Build history of the part. All positions in model axes, mm. A direction names the side the tool comes from. Give positions to 0.01 mm unless a question says otherwise; leave off trailing zeros. Loops run counter-clockwise (first coordinate to the right, second up) from the corner with the lowest first, then second, coordinate; pieces in that order, holes last. Notation, with made-up numbers: (78, 73) -> (106, 73) arc R26 ccw to (106, 96) -> close; hole circle Ø6 at (-29.75, -15.5). An arc over 180 degrees is marked (long way). Answer as a JSON object with one key per item and string values. Group by question number.
from build123d import *

# Parameters (mm, degrees)
SKETCH1_R           = 3
BOSS_EXTRUDE1_DEPTH = 7.5
SKETCH2_W           = 9
SKETCH2_H           = 5
CUT_EXTRUDE1_DEPTH  = 4.5
SKETCH3_W           = 5
SKETCH3_H           = 5
CUT_EXTRUDE2_DEPTH  = 1.5
CUT_EXTRUDE3_DEPTH  = 6


with BuildPart() as part:
    # Sketch1 → Boss-Extrude1 (new body)
    with BuildSketch(Plane.XY):
        with BuildLine():
            Line((-1.5, 5), (-3.5, 5))
            ThreePointArc((-3.5, 5), (-8.5, 0), (-3.5, -5))
            Line((-3.5, -5), (3.5, -5))
            Line((3.5, -5), (3.5, 5))
            Line((3.5, 5), (2.5, 5))
            Line((2.5, 5), (2.5, 4))
            Line((2.5, 4), (-1.5, 4))
            Line((-1.5, 4), (-1.5, 5))
        make_face()
        with Locations((-3.5, 0)):
            Circle(SKETCH1_R, mode=Mode.SUBTRACT)
    extrude(amount=BOSS_EXTRUDE1_DEPTH)

    # Sketch2 → Cut-Extrude1 (cut)
    with BuildSketch(Plane.XY.offset(7.5)):
        with Locations((-4, 2.5)):
            Rectangle(SKETCH2_W, SKETCH2_H)
    extrude(amount=-CUT_EXTRUDE1_DEPTH, mode=Mode.SUBTRACT)

    # Sketch3 → Cut-Extrude2 (cut)
    with BuildSketch(Plane.XY.offset(7.5)):
        with Locations((-6, -2.5)):
            Rectangle(SKETCH3_W, SKETCH3_H)
    extrude(amount=-CUT_EXTRUDE2_DEPTH, mode=Mode.SUBTRACT)

    # Sketch4 → Cut-Extrude3 (cut)
    with BuildSketch(Plane(origin=(0, 5, 0), x_dir=(1, 0, 0), z_dir=(0, 1, 0))):
        Polygon((3.5, -6.5), (2.5, -6.5), (0.5, -3), (0.5, -7.5), (3.5, -7.5), align=None)
    extrude(amount=-CUT_EXTRUDE3_DEPTH, mode=Mode.SUBTRACT)


solid = part.part
(1) Probe line 1 along X through (y, z) = (0, 2.5); line 2 along Z through (x, y) = (-2, 4); line 3 along Z through (x, y) = (-5, -3.5). List the from-to ranges inside material, lowest first. Write a range as [from, to].
(2) 3-axis set-ups, long thin cutter, end or side, ignore diameter. For faces 1 (the flat face through (3, 5, 3)), 2 (the flat face through (0.5, -0.5, 5.2)), 3 (the flat face through (-8, 0, 5)), 4 (the flat face through (-6, -2, 6)), 5 (the flat face through (1, 4, 2)): which of +Z, -Z, +X, -X, +Y, -Y reach the whole face in a straight line?
(3) Saw through at C-C on x = -2.25. List the corners of the cut face in (y, z), plus the area to 3 significant figures.
(4) Saw through at D-D on z = 6.75. List the corners of the cut face in (x, y), plus the area to 3 significant figures.
(5) Pull direction X, two halves, no side cores. Call faces 6 (the cylindrical face through (-2.116, -2.662, 2.864)), 7 (the flat face through (-3.5, -4, 7)), 8 (the flat face through (0, -3, 7.5)), 9 (the flat face through (3.5, 0, 4)): pulls with the +X half, pulls with the -X half, needs draft (parallel to the pull), parting line crosses it, or undercut.
(6) Saw through at B-B on y = 2. List the corners of the cut face in (x, z).
(7) Saw through at A-A on z = 2. List the corners of the cut face in (x, y), plus the area to 3 significant figures.
(8) Pin check, flat tips, straight feed: pin 1 (1.6 mm diameter, centred on x = -8, z = 5, fed in from +Y); pin 2 (3 mm diameter, centred on x = -6.5, z = 6, fed in from -Y); pin 3 (0.5 mm diameter, centred on x = 3, y = 1, fed in from +Z); pin 4 (2.5 mm diameter, centred on x = 2, z = 5, fed in from +Y). Stop position of each tip, or through.
Calculated:
{
 "1": {"line 1": "x = [-8.5, -6.5], [-0.5, 3.5]", "line 2": "z = [0, 3]", "line 3": "z = [0, 6]"},
 "2": {"face 1": "+Z, -Z, +X, -X, +Y", "face 2": "+Z, +Y", "face 3": "+Z, -X, +Y", "face 4": "+Z, -X, +Y, -Y", "face 5": "+Z, -Z, +Y"},
 "3": {"outline": "(-5, 0) -> (-2.73, 0) -> (-2.73, 7.5) -> (-5, 7.5) -> close; (2.73, 0) -> (5, 0) -> (5, 3) -> (2.73, 3) -> close", "area": "23.9 mm^2"},
 "4": {"outline": "(-3.5, -5) -> (3.5, -5) -> (3.5, -1) -> (0.5, -1) -> (0.5, 0) -> (-0.5, 0) arc R3 cw to (-3.5, -3) -> close", "area": "24.9 mm^2"},
 "5": {"face 6": "undercut", "face 7": "pulls with the -X half", "face 8": "needs draft", "face 9": "pulls with the +X half"},
 "6": {"outline": "(-8.08, 0) -> (-5.74, 0) -> (-5.74, 3) -> (-8.08, 3) -> close; (-1.26, 0) -> (3.5, 0) -> (3.5, 6.5) -> (2.5, 6.5) -> (0.5, 3) -> (-1.26, 3) -> close"},
 "7": {"outline": "(-3.5, -5) -> (3.5, -5) -> (3.5, 5) -> (2.5, 5) -> (2.5, 4) -> (-1.5, 4) -> (-1.5, 5) -> (-3.5, 5) arc R5 ccw to start; hole circle Ø6 at (-3.5, 0)", "area": "77.0 mm^2"},
 "8": {"pin 1": "stops at y = 0", "pin 2": "stops at y = -4.77", "pin 3": "stops at z = 6.5", "pin 4": "stops at y = 5"}
}
